Model file for the job. Use its own axes, mm. Give positions to 0.01 mm unless a question says otherwise; leave off trailing zeros. Write each loop counter-clockwise with the first axis right and the second up, starting at its lowest first coordinate (ties: lowest second). Pieces come first, ordered by that corner, then holes. Notation, with made-up numbers: (81, -5.5) - (93, -5.5) arc R18 ccw to (93, 3.5) - close; hole circle Ø10 at (37, 28). An arc over 180 degrees is marked (long way). One line per item, written item: value. Start each with the question number.
(1) Probe L1, parallel to X at y = -75, z = 27; L2, parallel to X at y = -58, z = -15; L3, parallel to Z at x = 47, y = -23. List the from-to ranges inside material, lowest first.
(2) Drop flat-ended pins along their axis: P1, Ø1.5, axis at x = 80.5, z = -58.5, coming from the +Y side; P2, Ø6, axis at y = -45, z = 19, coming from the +X side; P3, Ø4, axis at x = -79.5, y = -15.5, coming from the +Z side; P4, Ø3, axis at x = 27.5, y = -9.5, coming from the +Z side. Give the stop position or say it passes through.
(3) Mould opens along Z. For faces 1 (the face through (-43.93, -36.98, 3.37)), 2 (the face through (-40.2, -75.313, 34.039)), 3 (the face through (70.9, -79.7, 52.5)), 4 (the face through (115.274, -36.975, -20.597)) say: pulls with the +Z half, pulls with the -Z half, needs draft (parallel to the pull), parting line crosses it, or undercut.
(4) Cut at A-A, the plane y = -68. List the corners of the cut face in (x, z), and give its area (3 significant figures).
(5) Cut at B-B, the plane z = -71.5. List the corners of the cut face in (x, y), and give its area (3 significant figures).
from build123d import *

# Parameters (mm, degrees)
F1_DEPTH   = 80
F2_C1_SIZE = 5
F2_C2_SIZE = 5
F2_C3_SIZE = 5
F2_C4_SIZE = 5
F2_C5_SIZE = 5
F2_C6_SIZE = 5
F2_C7_SIZE = 5
F2_C8_SIZE = 5


with BuildPart() as f1:
    # F0 (on Front) → F1 (new body)
    with BuildSketch(Plane.XZ):
        with BuildLine():
            Line((0, 58.1298414463), (0, 81.0960731047))
            ThreePointArc((0, 81.0960731047), (-72.594350102, 57.0156445727), (-123.5749638583, 0))
            Line((-123.5749638583, 0), (-107.2012897506, -40.625271212))
            Line((-107.2012897506, -40.625271212), (-32.4384310855, -91.2910051649))
            Line((-32.4384310855, -91.2910051649), (0, -91.2910051649))
            Line((0, -91.2910051649), (0, -31.8701585537))
            ThreePointArc((0, -31.8701585537), (-45, 13.1298414463), (0, 58.1298414463))
        make_face()
        with BuildLine():
            ThreePointArc((123.5749638583, 0), (72.594350102, 57.0156445727), (0, 81.0960731047))
            Line((0, 81.0960731047), (0, 58.1298414463))
            ThreePointArc((0, 58.1298414463), (31.8198051534, 44.9496465997), (45, 13.1298414463))
            ThreePointArc((45, 13.1298414463), (31.8198051534, -18.6899637071), (0, -31.8701585537))
            Line((0, -31.8701585537), (0, -91.2910051649))
            Line((0, -91.2910051649), (32.4384310855, -91.2910051649))
            Line((32.4384310855, -91.2910051649), (107.2012897506, -40.625271212))
            Line((107.2012897506, -40.625271212), (123.5749638583, 0))
        make_face()
    extrude(amount=F1_DEPTH)

    # F2: chamfer of 5 on 8 edges, made by hand

    # F2_c1
    f2_c1_edges = [f1.edges().sort_by_distance(p)[0] for p in [
        (0, -80, -31.8701585537),
    ]]
    chamfer(f2_c1_edges, length=F2_C1_SIZE)

    # F2_c2
    f2_c2_edges = [f1.edges().sort_by_distance(p)[0] for p in [
        (-72.594350102, -80, 57.0156445727),
    ]]
    chamfer(f2_c2_edges, length=F2_C2_SIZE)

    # F2_c3
    f2_c3_edges = [f1.edges().sort_by_distance(p)[0] for p in [
        (-114.129610425, -80, -23.4351827451),
    ]]
    chamfer(f2_c3_edges, length=F2_C3_SIZE)

    # F2_c4
    f2_c4_edges = [f1.edges().sort_by_distance(p)[0] for p in [
        (-66.1115818198, -80, -68.4711862478),
    ]]
    chamfer(f2_c4_edges, length=F2_C4_SIZE)

    # F2_c5
    f2_c5_edges = [f1.edges().sort_by_distance(p)[0] for p in [
        (4.4563329797, -80, -91.2910051649),
    ]]
    chamfer(f2_c5_edges, length=F2_C5_SIZE)

    # F2_c6
    f2_c6_edges = [f1.edges().sort_by_distance(p)[0] for p in [
        (73.5088851707, -80, -63.4581381884),
    ]]
    chamfer(f2_c6_edges, length=F2_C6_SIZE)

    # F2_c7
    f2_c7_edges = [f1.edges().sort_by_distance(p)[0] for p in [
        (117.0626938618, -80, -16.1578111957),
    ]]
    chamfer(f2_c7_edges, length=F2_C7_SIZE)

    # F2_c8
    f2_c8_edges = [f1.edges().sort_by_distance(p)[0] for p in [
        (86.848352424, -80, 46.3883216842),
    ]]
    chamfer(f2_c8_edges, length=F2_C8_SIZE)


solid = f1.part
Answers follow:
1. L1: x = -105.97 to -42.81, 42.81 to 105.97
1. L2: x = -117.53 to -35.12, 35.12 to 117.53
1. L3: z = -81.42 to 70.45
2. P1: stops at y = 0
2. P2: stops at x = 114.16
2. P3: stops at z = 53.65
2. P4: stops at z = 77.21
3. face 1: undercut
3. face 2: undercut
3. face 3: pulls with the +Z half
3. face 4: pulls with the -Z half
4. outline: (-123.57, 0) - (-107.2, -40.63) - (-32.44, -91.29) - (32.44, -91.29) - (107.2, -40.63) - (123.57, 0) arc R148.5 ccw to (0, 81.1) arc R148.5 ccw to start; hole circle Ø90 at (0, 13.13)
4. area: 24,000 mm²
5. outline: (-61.64, -75) - (-52.73, -80) - (52.73, -80) - (61.64, -75) - (61.64, 0) - (-61.64, 0) - close
5. area: 9,820 mm²
